Could you check a few things on this model? Use its own coordinates, in mm. Face numbers are marked on the shaded views. A direction names the side the tool comes from. Give positions to 0.01 mm unless a question says otherwise; leave off trailing zeros. Loops run counter-clockwise (first coordinate to the right, second up) from the corner with the lowest first, then second, coordinate; pieces in that order, holes last.
1. I need wall thicknesses on line 1 along X through (y, z) = (177.5, 245.5); line 2 along Y through (x, z) = (-73.5, 225); line 3 along Z through (x, y) = (-97, -273.5). Which ranges of each line are inside material? Lowest first, please.
2. For the marked faces 1 and 2, which set-ups out of +Z, -Z, +X, -X, +Y, -Y let a thin tool reach every point of the face, with its end or its side?
3. Imagine slicing it at B-B (z = -148). List the corners of the cut face in (x, y) for me, plus the area to 3 significant figures.
4. Imagine slicing it at C-C (y = -283). List the corners of the cut face in (x, z) for me.
5. Imagine slicing it at A-A (x = -62). List the corners of the cut face in (y, z) for me, plus the area to 3 significant figures.
6. For P1, Ø5, axis at x = -71, y = -391.5, coming from the -Z side; P2, Ø12, axis at x = -50.5, y = -375.5, coming from the -Z side; P3, Ø8, axis at y = 243, z = -55.5, coming from the -X side, each with a flat end and sliding along its axis, tell me the tip position at first contact or that it passes through.
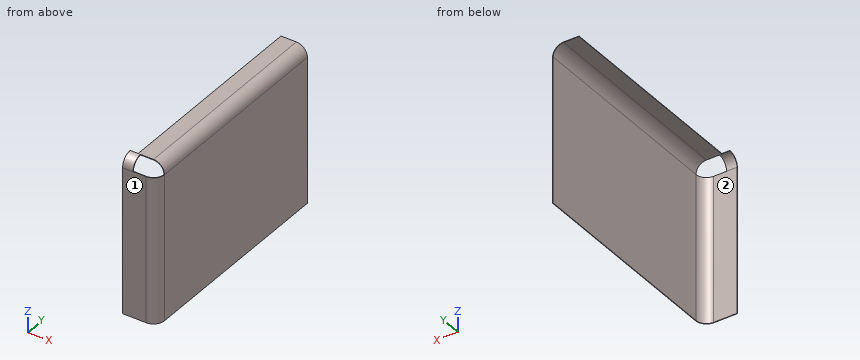
```python
from build123d import *

# Parameters (mm, degrees)
F0_W     = 1000
F0_H     = 700
F1_DEPTH = 3
F3_DEPTH = 1000
F5_DEPTH = 700
F7_DEPTH = 50


with BuildPart() as f1:
    # F0 (on Right) → F1 (new body)
    with BuildSketch(Plane.YZ):
        Rectangle(F0_W, F0_H)
    extrude(amount=F1_DEPTH)

    # F2 (on face) → F3 (join)
    with BuildSketch(Plane(origin=(0, 500, 0), x_dir=(-1, 0, 0), z_dir=(0, 1, 0))):
        with BuildLine():
            Line((123.797374, 403), (50, 403))
            ThreePointArc((50, 403), (12.523341, 387.476659), (-3, 350))
            Line((-3, 350), (0, 350))
            ThreePointArc((0, 350), (14.644661, 385.355339), (50, 400))
            Line((50, 400), (123.797374, 400))
            Line((123.797374, 400), (123.797374, 403))
        make_face()
    extrude(amount=-F3_DEPTH)

    # F4 (on face) → F5 (join)
    with BuildSketch(Plane(origin=(0, 0, -350), x_dir=(1, 0, 0), z_dir=(0, 0, -1))):
        with BuildLine():
            Line((-162.145862, 550), (-50, 550))
            ThreePointArc((-50, 550), (-14.644661, 535.355339), (0, 500))
            Line((0, 500), (3, 500))
            ThreePointArc((3, 500), (-12.523341, 537.476659), (-50, 553))
            Line((-50, 553), (-162.145862, 553))
            Line((-162.145862, 553), (-162.145862, 550))
        make_face()
    extrude(amount=-F5_DEPTH)

    # F6 (on face) → F7 (join)
    with BuildSketch(Plane(origin=(-162.145862, 0, 0), x_dir=(0, -1, 0), z_dir=(-1, 0, 0))):
        with BuildLine():
            Line((500, 403), (500, 400))
            ThreePointArc((500, 400), (535.355339, 385.355339), (550, 350))
            Line((550, 350), (553, 350))
            ThreePointArc((553, 350), (537.476659, 387.476659), (500, 403))
        make_face()
    extrude(amount=-F7_DEPTH)


solid = f1.part
```
Derived:
1. line 1: x = 0 to 3
1. line 2: y = -553 to -550
1. line 3: z = 400 to 403
2. face 1: +Z, -Z, +X, -X, -Y
2. face 2: -Z, -X, +Y
3. outline: (-162.15, -553) - (-50, -553) arc R53 ccw to (3, -500) - (3, 500) - (0, 500) - (0, -500) arc R50 cw to (-50, -550) - (-162.15, -550) - close
3. area: 3,580 mm2
4. outline: (-123.8, 400) - (-50, 400) arc R50 cw to (0, 350) - (0, -350) - (3, -350) - (3, 350) arc R53 ccw to (-50, 403) - (-123.8, 403) - close
5. outline: (-553, -350) - (-550, -350) - (-550, 350) - (-553, 350) - close; (-500, 400) - (500, 400) - (500, 403) - (-500, 403) - close
5. area: 5,100 mm2
6. P1: stops at z = 400
6. P2: stops at z = 399.7
6. P3: stops at x = 0
